from build123d import *

# Parameters (mm, degrees)
BOSS_EXTRUDE1_DEPTH = 740
CUT_EXTRUDE1_REACH  = 742.54
SKETCH2_R           = 1.5
CUT_EXTRUDE2_REACH  = 742.54
SKETCH3_R           = 1.5


with BuildPart() as part:
    # Sketch1 → Boss-Extrude1 (new body)
    with BuildSketch(Plane(origin=(0, 0, 0), x_dir=(0, 0, -1), z_dir=(1, 0, 0))):
        Polygon((0, 0), (0, 20), (1, 20), (1, 1), (20, 1), (20, 0), align=None)
    extrude(amount=BOSS_EXTRUDE1_DEPTH)

    # Sketch2 → Cut-Extrude1 (cut, up to next)
    with BuildSketch(Plane.XY, mode=Mode.PRIVATE) as cut_extrude1_sk1:
        with Locations((10, 10)):
            Circle(SKETCH2_R)
    cut_extrude1_tool1 = extrude(cut_extrude1_sk1.sketch, amount=-CUT_EXTRUDE1_REACH, mode=Mode.PRIVATE) & part.part
    # Sketch2 → Cut-Extrude1 (cut, up to next)
    with BuildSketch(Plane.XY, mode=Mode.PRIVATE) as cut_extrude1_sk2:
        with Locations((730, 10)):
            Circle(SKETCH2_R)
    cut_extrude1_tool2 = extrude(cut_extrude1_sk2.sketch, amount=-CUT_EXTRUDE1_REACH, mode=Mode.PRIVATE) & part.part
    add(cut_extrude1_tool1.solids().sort_by_distance((10, 10, 0))[0], mode=Mode.SUBTRACT)
    add(cut_extrude1_tool2.solids().sort_by_distance((730, 10, 0))[0], mode=Mode.SUBTRACT)

    # Sketch3 → Cut-Extrude2 (cut, up to next)
    with BuildSketch(Plane.XZ, mode=Mode.PRIVATE) as cut_extrude2_sk1:
        with Locations(Location((10, -10, 0), (0, 0, 270))):
            Circle(SKETCH3_R)
    cut_extrude2_tool1 = extrude(cut_extrude2_sk1.sketch, amount=-CUT_EXTRUDE2_REACH, mode=Mode.PRIVATE) & part.part
    # Sketch3 → Cut-Extrude2 (cut, up to next)
    with BuildSketch(Plane.XZ, mode=Mode.PRIVATE) as cut_extrude2_sk2:
        with Locations(Location((730, -10, 0), (0, 0, 270))):
            Circle(SKETCH3_R)
    cut_extrude2_tool2 = extrude(cut_extrude2_sk2.sketch, amount=-CUT_EXTRUDE2_REACH, mode=Mode.PRIVATE) & part.part
    add(cut_extrude2_tool1.solids().sort_by_distance((10, 0, -10))[0], mode=Mode.SUBTRACT)
    add(cut_extrude2_tool2.solids().sort_by_distance((730, 0, -10))[0], mode=Mode.SUBTRACT)


solid = part.part
Read the model definition and answer for the solid it produces. Units are mm, in the model's axes. A direction names the side the tool comes from. Give positions to 0.01 mm unless a question says otherwise; leave off trailing zeros. Write each loop counter-clockwise with the first axis right and the second up, starting at its lowest first coordinate (ties: lowest second). Pieces come first, ordered by that corner, then holes. Notation, with made-up numbers: (66.5, -35.75) - (94.5, -35.75) arc R21 cw to (94.5, -31.75) - close; hole circle Ø1 at (67.5, 88.5). An arc over 180 degrees is marked (long way). Return JSON: item names as keys, results as strings.
Q1. A cutting plane is placed at C-C, the plane z = -14.5. Determine the outline of the cut face in (x, y).
Reply:
{"outline": "(0, 0) - (740, 0) - (740, 1) - (0, 1) - close"}
Q2. Consider line 1 along X through (y, z) = (0.6, -10); line 2 along Y through (x, z) = (730, -0.35); line 3 along Z through (x, y) = (168.5, 17). Determine where each line is inside the solid, lowest interval first. Write a range as [from, to].
Reply:
{"line 1": "[0, 8.5], [11.5, 728.5], [731.5, 740]", "line 2": "[0, 8.5], [11.5, 20]", "line 3": "[-1, 0]"}
Q3. For faces 1 (the face through (740, 0.4, -5.6)), 2 (the face through (365, 11, -1)), determine the directions among +Z, -Z, +X, -X, +Y, -Y from which every point of the face is accessible in a straight line to the end or side of a thin tool.
Reply:
{"face 1": "+Z, -Z, +X, +Y, -Y", "face 2": "-Z, +X, -X, +Y"}
Q4. A cutting plane is placed at B-B, the plane y = 16.75. Determine the outline of the cut face in (x, z), and give its area (3 significant figures).
Reply:
{"outline": "(0, -1) - (740, -1) - (740, 0) - (0, 0) - close", "area": "740 mm²"}
Q5. A cutting plane is placed at A-A, the plane x = 340. Determine the outline of the cut face in (y, z).
Reply:
{"outline": "(0, -20) - (1, -20) - (1, -1) - (20, -1) - (20, 0) - (0, 0) - close"}
Q6. For a pull along Y with two mould halves and no side action, classify faces 3 (the face through (365, 1, -10)), 4 (the face through (365, 0, -10)), 5 (the face through (365, 10, 0)) as released by +Y, released by -Y, zero draft, split by the parting line, or undercut.
Reply:
{"face 3": "released by +Y", "face 4": "released by -Y", "face 5": "zero draft"}
Q7. Given P1, Ø2, axis at x = 424.5, z = -8, coming from the +Y side; P2, Ø3, axis at x = 75, y = 5.5, coming from the -Z side; P3, Ø2.5, axis at x = 730, y = 10, coming from the +Z side, each flat-ended and moving along its own axis, determine where each tip first touches the part or whether it passes through.
Reply:
{"P1": "y = 1", "P2": "z = -1", "P3": "through"}
